Build history of the part. All positions in model axes, mm. Give positions to 0.01 mm unless a question says otherwise; leave off trailing zeros. Write each loop counter-clockwise with the first axis right and the second up, starting at its lowest first coordinate (ties: lowest second). Pieces come first, ordered by that corner, then holes. Notation, with made-up numbers: (61.5, 4.5) -> (92.5, 4.5) arc R14 ccw to (92.5, 25.5) -> close; hole circle Ø1 at (86, -29.5). An arc over 180 degrees is marked (long way). Put each result on its own line as item: value.
from build123d import *

# Parameters (mm, degrees)
SKETCH3_W                                    = 431.251100871
SKETCH3_H                                    = 25.4
EXTRUDE1_DEPTH                               = 6.35
CSK_FOR_5_16_FLAT_HEAD_SOCKET_CAP_SC_2_COUNT = 2
CSK_FOR_5_16_FLAT_HEAD_SOCKET_CAP_SC_2_PITCH = 411.312205256


with BuildPart() as part:
    # Sketch3 → Extrude1 (new body)
    with BuildSketch(Plane(origin=(0, 0, 0), x_dir=(-1, 0, 0), z_dir=(0, 0, -1))):
        with Locations((-0.444447807, -41.102479446)):
            Rectangle(SKETCH3_W, SKETCH3_H)
    extrude(amount=EXTRUDE1_DEPTH)

    # Sketch4 → CSK for 5/16 Flat Head Socket Cap Screw1 (revolve, cut)
    with BuildSketch(Plane(origin=(205.656102628, -41.102479446, -6.35), x_dir=(0, 1, 0), z_dir=(1, 0, 0))):
        Polygon((0, 0), (0, 6.35), (4.1021, 6.35), (4.1021, 5.373016172), (8.7727917, 0), align=None)
    csk_for_5_16_flat_head_socket_cap_screw1 = revolve(axis=Axis((205.656102628, -41.102479446, -12.7), (0, 0, 1)), mode=Mode.SUBTRACT)

    # CSK for 5_16 Flat Head Socket Cap Sc 2: CSK for 5/16 Flat Head Socket Cap Screw1 ×2
    with Locations(*[(-i * CSK_FOR_5_16_FLAT_HEAD_SOCKET_CAP_SC_2_PITCH, 0, 0) for i in range(1, CSK_FOR_5_16_FLAT_HEAD_SOCKET_CAP_SC_2_COUNT)]):
        add(csk_for_5_16_flat_head_socket_cap_screw1, mode=Mode.SUBTRACT)


solid = part.part
1) Wall check: L1, parallel to X at y = -46, z = -3.75; L2, parallel to X at y = -40.5, z = -2.75 (3 decimals). Give the ranges that are in metal, low to high.
Filled sheet:
L1: -215.18 to -209.95, -201.36 to 201.36, 209.95 to 216.07
L2: -215.181 to -211.267, -200.045 to 200.045, 211.267 to 216.07
2) Slice it at A-A (z = -3.75). Write the cut outline in (x, y).
Filled sheet:
outline: (-215.18, -53.8) -> (216.07, -53.8) -> (216.07, -28.4) -> (-215.18, -28.4) -> close; hole circle Ø13.03 at (-205.66, -41.1); hole circle Ø13.03 at (205.66, -41.1)
3) Pin check, flat tips, straight feed: pin 1 (5 mm diameter, centred on x = 166.5, y = -42, fed in from +Z); pin 2 (5 mm diameter, centred on x = -205.66, y = -41.1, fed in from -Z). Stop position of each tip, or through.
Filled sheet:
pin 1: z = 0
pin 2: through
4) Pull direction X, two halves, no side cores. Call faces 1 (the flat face through (3, -41, 0)), 2 (the cylindrical face through (209.66, -41.99, -0.5)): released by +X, released by -X, zero draft, split by the parting line, or undercut.
Filled sheet:
face 1: zero draft
face 2: undercut
